from build123d import *

# Parameters (mm, degrees)
SKETCH1_W                                    = 68
SKETCH1_H                                    = 68
BOSS_EXTRUDE1_DEPTH                          = 20
CUT_EXTRUDE1_REACH                           = 54.077
SKETCH2_R                                    = 5
SKETCH3_R                                    = 6.5
CUT_EXTRUDE2_DEPTH                           = 5
CHAMFER2_SIZE                                = 0.5
CHAMFER4_SIZE                                = 0.5
CHAMFER5_SIZE                                = 0.25
CBORE_FOR_M8_HEX_SOCKET_HEAD_CAP_SCR_2_COUNT = 2
CBORE_FOR_M8_HEX_SOCKET_HEAD_CAP_SCR_2_PITCH = 59.39696962
F_8_0MM_DOWEL_HOLE1_AT_2_COUNT               = 2
F_8_0MM_DOWEL_HOLE1_AT_2_PITCH               = 59.39696962


with BuildPart() as part:
    # Sketch1 → Boss-Extrude1 (new body)
    with BuildSketch(Plane(origin=(0, 0, 0), x_dir=(1, 0, 0), z_dir=(0, 1, 0))):
        Rectangle(SKETCH1_W, SKETCH1_H)
    extrude(amount=-BOSS_EXTRUDE1_DEPTH)

    # Sketch2 → Cut-Extrude1 (cut, up to next)
    with BuildSketch(Plane(origin=(0, 0, 0), x_dir=(1, 0, 0), z_dir=(0, 1, 0)), mode=Mode.PRIVATE) as cut_extrude1_sk1:
        with Locations(Location((-19, 0, 0), (0, 0, 270))):
            Circle(SKETCH2_R)
    cut_extrude1_tool1 = extrude(cut_extrude1_sk1.sketch, amount=-CUT_EXTRUDE1_REACH, mode=Mode.PRIVATE) & part.part
    # Sketch2 → Cut-Extrude1 (cut, up to next)
    with BuildSketch(Plane(origin=(0, 0, 0), x_dir=(1, 0, 0), z_dir=(0, 1, 0)), mode=Mode.PRIVATE) as cut_extrude1_sk2:
        with Locations(Location((19, 0, 0), (0, 0, 270))):
            Circle(SKETCH2_R)
    cut_extrude1_tool2 = extrude(cut_extrude1_sk2.sketch, amount=-CUT_EXTRUDE1_REACH, mode=Mode.PRIVATE) & part.part
    add(cut_extrude1_tool1.solids().sort_by_distance((-19, 0, 0))[0], mode=Mode.SUBTRACT)
    add(cut_extrude1_tool2.solids().sort_by_distance((19, 0, 0))[0], mode=Mode.SUBTRACT)

    # Sketch3 → Cut-Extrude2 (cut)
    with BuildSketch(Plane(origin=(0, 0, 0), x_dir=(1, 0, 0), z_dir=(0, 1, 0))):
        with Locations(Location((-19, 0, 0), (0, 0, 270))):
            Circle(SKETCH3_R)
        with Locations(Location((19, 0, 0), (0, 0, 270))):
            Circle(SKETCH3_R)
    extrude(amount=-CUT_EXTRUDE2_DEPTH, mode=Mode.SUBTRACT)

    # Chamfer2
    chamfer2_edges = [part.edges().sort_by_distance(p)[0] for p in [
        (-34, -20, 0),
        (0, -20, 34),
        (34, -20, 0),
        (0, 0, 34),
        (-34, 0, 0),
        (0, 0, -34),
        (34, 0, 0),
        (34, -10, 34),
        (-34, -10, 34),
        (-34, -10, -34),
        (34, -10, -34),
        (0, -20, -34),
    ]]
    chamfer(chamfer2_edges, length=CHAMFER2_SIZE)

    # Chamfer4
    chamfer4_edges = [part.edges().sort_by_distance(p)[0] for p in [
        (-19, 0, -6.5),
        (19, 0, -6.5),
    ]]
    chamfer(chamfer4_edges, length=CHAMFER4_SIZE)

    # Chamfer5
    chamfer5_edges = [part.edges().sort_by_distance(p)[0] for p in [
        (-19, -20, -5),
        (19, -20, -5),
        (-19, -5, -5),
        (19, -5, -5),
    ]]
    chamfer(chamfer5_edges, length=CHAMFER5_SIZE)

    # Sketch5 → CBORE for M8 Hex Socket Head Cap Screw1 (revolve, cut)
    with BuildSketch(Plane(origin=(-21, -20, 21), x_dir=(0, 0, -1), z_dir=(1, 0, 0))):
        Polygon((0, 0), (0, 20), (4.525, 20), (4.5, 19.975), (4.5, 8.6), (7.5, 8.6), (7.5, 0.025), (7.525, 0), align=None)
    cbore_for_m8_hex_socket_head_cap_screw1 = revolve(axis=Axis((-21, -26.35, 21), (0, 1, 0)), mode=Mode.SUBTRACT)

    # CBORE for M8 Hex Socket Head Cap Scr 2: CBORE for M8 Hex Socket Head Cap Screw1 ×2
    with Locations(*[Vector(0.7071067811865476, 0, -0.7071067811865476) * (i * CBORE_FOR_M8_HEX_SOCKET_HEAD_CAP_SCR_2_PITCH) for i in range(1, CBORE_FOR_M8_HEX_SOCKET_HEAD_CAP_SCR_2_COUNT)]):
        add(cbore_for_m8_hex_socket_head_cap_screw1, mode=Mode.SUBTRACT)

    # Sketch7 → Ø8.0mm Dowel Hole1 (revolve, cut)
    with BuildSketch(Plane(origin=(-21, -20, -21), x_dir=(0, 0, -1), z_dir=(1, 0, 0))):
        Polygon((0, 0), (0, 20), (4.025, 20), (4, 19.975), (4, 0.025), (4.025, 0), align=None)
    f_8_0mm_dowel_hole1 = revolve(axis=Axis((-21, -26.35, -21), (0, 1, 0)), mode=Mode.SUBTRACT)

    # Ø8.0mm Dowel Hole1 at 2: Ø8.0mm Dowel Hole1 ×2
    with Locations(*[Vector(0.7071067811865476, 0, 0.7071067811865476) * (i * F_8_0MM_DOWEL_HOLE1_AT_2_PITCH) for i in range(1, F_8_0MM_DOWEL_HOLE1_AT_2_COUNT)]):
        add(f_8_0mm_dowel_hole1, mode=Mode.SUBTRACT)


solid = part.part
Read the model definition and answer for the solid it produces. Units are mm, in the model's axes. A direction names the side the tool comes from. Give positions to 0.01 mm unless a question says otherwise; leave off trailing zeros. Write each loop counter-clockwise with the first axis right and the second up, starting at its lowest first coordinate (ties: lowest second). Pieces come first, ordered by that corner, then holes. Notation, with made-up numbers: (88.25, -32.75) -> (145.25, -32.75) arc R21 cw to (145.25, -28.75) -> close; hole circle Ø1 at (36, -28). An arc over 180 degrees is marked (long way). Answer as a JSON object with one key per item and string values. Group by question number.
1) Each of these flat-tipped pins is pushed along its axis until it touches: P1, Ø4, axis at x = 20.5, z = -3, coming from the +Y side; P2, Ø12, axis at x = -21, z = 21, coming from the -Y side. Where does it stop, or does it pass through?
2) The mould has two halves that part along Z. Classify faces 1 (the flat face through (0, -20, 0)), 2 (the flat face through (0, -10, -34)), 3 (the flat face through (-21, -11.4, 26)): +Z half, -Z half, draft (parallel to the pull), parting line (faces both ways), or undercut.
3) Find section B-B (y = -12.25). Write down the section's boundary in (x, z).
4) A tool of negligible diameter and unlimited length cuts with its end or side. For faces 4 (the cylindrical face through (25.445, -2.718, -0.846)), 5 (the cylindrical face through (27.654, -15.748, -24.461)), 6 (the cylindrical face through (-23.88, -12.4, -1.08)), from which of +Z, -Z, +X, -X, +Y, -Y can it reach the whole face along a straight path? Write none if from no direction.
5) Consider L1, parallel to X at y = -3.75, z = -21; L2, parallel to X at y = -13.75, z = 21; L3, parallel to Z at x = -23, y = -1. Determine where each line is inside the solid, lowest interval first. Write a range as from..to.
6) Find section A-A (z = -21). Write down the section's boundary in (x, y) (3 decimals), and give its area (3 significant figures).
7) Find section C-C (y = -6.25). Write down the section's boundary in (x, z), and give its area (3 significant figures).
8) Find section D-D (x = 21). Count the separate pieces of the cut face and the enclosed holes in it, and give its area (3 significant figures).
Values follow:
{
 "1": {"P1": "stops at y = -5", "P2": "stops at y = -11.4"},
 "2": {"face 1": "draft", "face 2": "-Z half", "face 3": "undercut"},
 "3": {"outline": "(-34, -33.5) -> (-33.5, -34) -> (33.5, -34) -> (34, -33.5) -> (34, 33.5) -> (33.5, 34) -> (-33.5, 34) -> (-34, 33.5) -> close; hole circle Ø15 at (-21, 21); hole circle Ø8 at (-21, -21); hole circle Ø10 at (-19, 0); hole circle Ø15 at (21, -21); hole circle Ø10 at (19, 0); hole circle Ø8 at (21, 21)"},
 "4": {"face 4": "+Y", "face 5": "-Y", "face 6": "+Y, -Y"},
 "5": {"L1": "x = -34..-25, -17..16.5, 25.5..34", "L2": "x = -34..-28.5, -13.5..17, 25..34", "L3": "z = -34..-24.46, -17.54..-5.12, 5.12..16.97, 25.03..34"},
 "6": {"outline": "(-34, -19.5) -> (-33.5, -20) -> (-25.025, -20) -> (-25, -19.975) -> (-25, -0.025) -> (-25.025, 0) -> (-33.5, 0) -> (-34, -0.5) -> close; (-17, -19.975) -> (-16.975, -20) -> (13.475, -20) -> (13.5, -19.975) -> (13.5, -11.4) -> (16.5, -11.4) -> (16.5, -0.025) -> (16.475, 0) -> (-16.975, 0) -> (-17, -0.025) -> close; (25.5, -11.4) -> (28.5, -11.4) -> (28.5, -19.975) -> (28.525, -20) -> (33.5, -20) -> (34, -19.5) -> (34, -0.5) -> (33.5, 0) -> (25.525, 0) -> (25.5, -0.025) -> close", "area": "968 mm2"},
 "7": {"outline": "(-34, -33.5) -> (-33.5, -34) -> (33.5, -34) -> (34, -33.5) -> (34, 33.5) -> (33.5, 34) -> (-33.5, 34) -> (-34, 33.5) -> close; hole circle Ø9 at (-21, 21); hole circle Ø8 at (-21, -21); hole circle Ø10 at (-19, 0); hole circle Ø10 at (19, 0); hole circle Ø9 at (21, -21); hole circle Ø8 at (21, 21)", "area": "4,240 mm2"},
 "8": {"separate pieces": "4", "enclosed holes": "0", "area": "768 mm2"}
}
